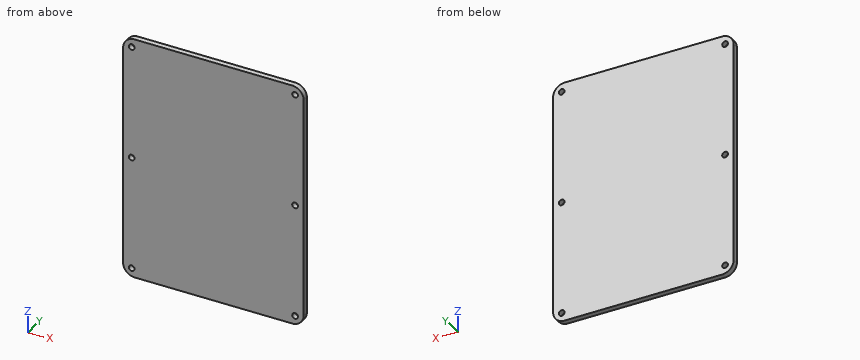
from build123d import *

# Parameters (mm, degrees)
SKETCH1_W               = 95
SKETCH1_H               = 127
BOSS_EXTRUDE1_DEPTH     = 3
FILLET1_R               = 6
SKETCH2_R               = 1.5
CUT_EXTRUDE1_DEPTH      = 80.35678925
LPATTERN2_COUNT         = 2
LPATTERN2_PITCH         = 59
MIRROR2_COPY_1_SKETCH_R = 1.5
MIRROR2_COPY_1_DEPTH    = 80.35678925
MIRROR2_COPY_2_SKETCH_R = 1.5
MIRROR2_COPY_2_DEPTH    = 80.35678925


with BuildPart() as part:
    # Sketch1 → Boss-Extrude1 (new body)
    with BuildSketch(Plane(origin=(0, 0, 0), x_dir=(1, 0, 0), z_dir=(0, 1, 0))):
        Rectangle(SKETCH1_W, SKETCH1_H)
    extrude(amount=BOSS_EXTRUDE1_DEPTH)

    # Fillet1
    fillet1_edges = [part.edges().sort_by_distance(p)[0] for p in [
        (47.5, 1.5, 63.5),
        (-47.5, 1.5, 63.5),
        (-47.5, 1.5, -63.5),
        (47.5, 1.5, -63.5),
    ]]
    fillet(fillet1_edges, radius=FILLET1_R)

    # Sketch2 → Cut-Extrude1 (cut, through all)
    with BuildSketch(Plane(origin=(0, 3, 0), x_dir=(1, 0, 0), z_dir=(0, 1, 0))):
        with Locations(Location((-43, 59, 0), (0, 0, 270))):
            Circle(SKETCH2_R)
    cut_extrude1 = extrude(amount=-CUT_EXTRUDE1_DEPTH, mode=Mode.SUBTRACT)

    # Mirror1: Cut-Extrude1 across plane
    add(cut_extrude1.mirror(Plane.XY), mode=Mode.SUBTRACT)

    # LPattern2: Cut-Extrude1 ×2
    with Locations(*[(0, 0, i * LPATTERN2_PITCH) for i in range(1, LPATTERN2_COUNT)]):
        add(cut_extrude1, mode=Mode.SUBTRACT)

    # Mirror2: Cut-Extrude1 across plane
    add(cut_extrude1.mirror(Plane(origin=(0, 0, 0), x_dir=(0, 0, 1), z_dir=(1, 0, 0))), mode=Mode.SUBTRACT)

    # Mirror2 copy 1 sketch → Mirror2 copy 1 (cut, through all)
    with BuildSketch(Plane(origin=(0, 3, 0), x_dir=(-1, 0, 0), z_dir=(0, 1, 0))):
        with Locations(Location((-43, 59, 0), (0, 0, 270))):
            Circle(MIRROR2_COPY_1_SKETCH_R)
    extrude(amount=-MIRROR2_COPY_1_DEPTH, mode=Mode.SUBTRACT)

    # Mirror2 copy 2 sketch → Mirror2 copy 2 (cut, through all)
    with BuildSketch(Plane(origin=(0, 3, 59), x_dir=(-1, 0, 0), z_dir=(0, 1, 0))):
        with Locations((-43, -59)):
            Circle(MIRROR2_COPY_2_SKETCH_R)
    extrude(amount=-MIRROR2_COPY_2_DEPTH, mode=Mode.SUBTRACT)


solid = part.part
The listing builds one solid part. Answer for the finished solid, in the listing's coordinates (mm). Give positions to 0.01 mm unless a question says otherwise; leave off trailing zeros. Write each loop counter-clockwise with the first axis right and the second up, starting at its lowest first coordinate (ties: lowest second). Pieces come first, ordered by that corner, then holes.
Item 1: Section A-A, the plane x = -43 is taken. Write down the section's boundary in (y, z), plus the area to 3 significant figures.
Item 2: Find the intervals of material crossed by line 1 along X through (y, z) = (1.4, -59); line 2 along Z through (x, y) = (43, 0.75), in increasing order.
Item 3: Section B-B, the plane z = -59 is taken. Write down the section's boundary in (x, y).
Completed:
1. outline: (0, -63.31) - (3, -63.31) - (3, -60.5) - (0, -60.5) - close; (0, -57.5) - (3, -57.5) - (3, -1.5) - (0, -1.5) - close; (0, 1.5) - (3, 1.5) - (3, 57.5) - (0, 57.5) - close; (0, 60.5) - (3, 60.5) - (3, 63.31) - (0, 63.31) - close
1. area: 353 mm2
2. line 1: x = -47.31 to -44.5, -41.5 to 41.5, 44.5 to 47.31
2. line 2: z = -63.31 to -60.5, -57.5 to -1.5, 1.5 to 57.5, 60.5 to 63.31
3. outline: (-47.31, 0) - (-44.5, 0) - (-44.5, 3) - (-47.31, 3) - close; (-41.5, 0) - (41.5, 0) - (41.5, 3) - (-41.5, 3) - close; (44.5, 0) - (47.31, 0) - (47.31, 3) - (44.5, 3) - close
